Autodesk Inventor part; units mm, degrees
ref_plane "YZ Plane" through (0, 0, 0) normal (1, 0, 0) x (0, 1, 0)
ref_plane "XZ Plane" through (0, 0, 0) normal (0, 1, 0) x (-1, 0, 0)
ref_plane "XY Plane" through (0, 0, 0) normal (0, 0, 1) x (1, 0, 0)
sketch "Эскиз1" plane through (0, 0, 0) normal (0, 0, 1) x (1, 0, 0)
  line L0 (-1.0718, 4) -> (83.0251, 4)
  circle A0 centre (14.7479, 10) radius 2
  circle A1 centre (62.7479, 10) radius 2
  line L1 (-1.0718, 4) -> (-3.896, 14.54)
  line L2 (83.0251, 4) -> (83.0251, 48.71)
  line L3 (-3.896, 14.54) -> (-6.6159, 24.6909)
  line L4 (-6.6159, 24.6909) -> (83.0251, 48.71)
  dimension "d0" = 10.509
extrude "Выдавливание1" add sketch "Эскиз1" along normal blind 4
sketch "Эскиз2" plane through (83.0251, 4, 0) normal (1, 0, 0) x (0, 0, -1)
  line L0 (-4, 0) -> (-4, 44.71)
  line L1 (-4, 44.71) -> (0, 44.71)
  line L2 (0, 44.71) -> (0, 40.71)
  line L3 (0, 40.71) -> (-4, 40.71)
  line L4 (-4, 40.71) -> (-4, 44.71)
  point P0 (0, -4)
  point P1 (-4, 40.71)
  dimension "d3" = 4
  dimension "d4" = 4
extrude "Выдавливание2" add sketch "Эскиз2" along normal blind 4
pattern_linear "Прямоуг.массив1" count 6 spacing 8 along (0, -1, 0) of "Выдавливание2"
sketch "Эскиз3" plane through (0, 0, 4) normal (0, 0, 1) x (1, 0, 0)
  circle A0 centre (56.9359, 33.9549) radius 2
  line L0 (-6.6159, 24.6909) -> (-1.0718, 4)
  line L1 (-1.0718, 4) -> (83.0251, 4)
  line L2 (83.0251, 4) -> (83.0251, 4.71)
  line L3 (83.0251, 4.71) -> (87.0251, 4.71)
  line L4 (87.0251, 8.71) -> (87.0251, 4.71)
  line L5 (83.0251, 8.71) -> (87.0251, 8.71)
  line L6 (83.0251, 8.71) -> (83.0251, 12.71)
  line L7 (83.0251, 12.71) -> (87.0251, 12.71)
  line L8 (87.0251, 16.71) -> (87.0251, 12.71)
  line L9 (83.0251, 16.71) -> (87.0251, 16.71)
  line L10 (83.0251, 16.71) -> (83.0251, 20.71)
  line L11 (83.0251, 20.71) -> (87.0251, 20.71)
  line L12 (87.0251, 24.71) -> (87.0251, 20.71)
  line L13 (83.0251, 24.71) -> (87.0251, 24.71)
  line L14 (83.0251, 24.71) -> (83.0251, 28.71)
  line L15 (83.0251, 28.71) -> (87.0251, 28.71)
  line L16 (87.0251, 32.71) -> (87.0251, 28.71)
  line L17 (83.0251, 32.71) -> (87.0251, 32.71)
  line L18 (83.0251, 32.71) -> (83.0251, 36.71)
  line L19 (83.0251, 36.71) -> (87.0251, 36.71)
  line L20 (87.0251, 40.71) -> (87.0251, 36.71)
  line L21 (83.0251, 40.71) -> (87.0251, 40.71)
  line L22 (83.0251, 40.71) -> (83.0251, 44.71)
  line L23 (83.0251, 44.71) -> (87.0251, 44.71)
  line L24 (87.0251, 48.71) -> (87.0251, 44.71)
  line L25 (83.0251, 48.71) -> (87.0251, 48.71)
  line L26 (83.0251, 48.71) -> (-6.6159, 24.6909)
  circle A1 centre (62.7479, 10) radius 2
  circle A2 centre (14.7479, 10) radius 2
  circle A3 centre (37.6174, 28.7785) radius 2
  point P0 (0, 0)
  point P1 (0, 0)
extrude "Выдавливание3" cut sketch "Эскиз3" against normal blind 10 contours A0 | A3
properties part number "KB33-046-004-009 - Передняя левая боковая пластина"
Here's how the part is built. I have some questions about the finished solid (model axes, mm). A direction names the side the tool comes from. Give positions to 0.01 mm unless a question says otherwise; leave off trailing zeros. Order: outer loops, then holes, each group sorted by start corner. A loop starts at its lowest first (then second) coordinate and runs counter-clockwise, first axis right, second up. Notation, with made-up numbers: M 79.5,-8 L 137.5,-8 A17 cw 137.5,0 Z; hole C 44.5,-24.75 d8. An arc over 180 degrees is marked long. Use a Markdown table: item, result. Add a question column.
1. On a 3-axis mill with a long thin cutter (end or side, diameter ignored), from which of +Z, -Z, +X, -X, +Y, -Y can I reach the whole of each face in a straight line? I mean faces 1 (the flat face through (83.025, 35, 2)), 2 (the flat face through (85, 4.71, 2)), 3 (the flat face through (37.577, 36.532, 1.972)). Say none if no direction works.
2. Suppose I cut it at C-C (x = 36.5). List the corners of the cut face in (y, z) for me, and give its area (3 significant figures).
3. I need wall thicknesses on probe 1 along X at (y, z) = (9, 0.3); probe 2 along Y at (x, z) = (37, 2.2); probe 3 along Y at (x, z) = (38, 0.95). Which ranges of each line are inside material? Lowest first, please. Write a range as from..to.
4. If we mould it in two halves opening along Y, with no side actions, what happens to faces 4 (the flat face through (87.025, 31, 2)), 5 (the flat face through (85, 32.71, 2)), 6 (the flat face through (40, 4, 2))? For each: +Y half, -Y half, draft (parallel to the pull), parting line (faces both ways), or undercut.
5. For pin 1 Ø1.2 at (x, z) = (84.5, 2) entering from -Y; pin 2 Ø3 at (x, y) = (56.94, 33.95) entering from -Z; pin 3 Ø2 at (y, z) = (27.5, 1.5) entering from +X, each with a flat end and sliding along its axis, tell me the tip position at first contact or that it passes through.
6. Suppose I cut it at A-A (y = 10). List the corners of the cut face in (x, z) for me, and give its area (3 significant figures).
7. Suppose I cut it at D-D (y = 35). List the corners of the cut face in (x, z) for me.
8. Suppose I cut it at B-B (z = 0.95). Give the number of separate pieces and of enclosed holes in the cut face, and give its area (3 significant figures).
Results list:
| question | item | result |
|---|---|---|
| 1 | face 1 | +Z, -Z, +X |
| 1 | face 2 | +Z, -Z, +X, -Y |
| 1 | face 3 | +Z, -Z, -X, +Y |
| 2 | outline | M 4,0 L 27.12,0 L 27.12,4 L 4,4 Z; M 30.44,0 L 36.24,0 L 36.24,4 L 30.44,4 Z |
| 2 | area | 116 mm² |
| 3 | probe 1 | x = -2.41..13.02, 16.48..61.02, 64.48..83.03 |
| 3 | probe 2 | y = 4..26.88, 30.68..36.38 |
| 3 | probe 3 | y = 4..26.82, 30.74..36.65 |
| 4 | face 4 | draft |
| 4 | face 5 | undercut |
| 4 | face 6 | -Y half |
| 5 | pin 1 | stops at y = 4.71 |
| 5 | pin 2 | passes through |
| 5 | pin 3 | stops at x = 83.03 |
| 6 | outline | M -2.68,0 L 12.75,0 L 12.75,4 L -2.68,4 Z; M 16.75,0 L 60.75,0 L 60.75,4 L 16.75,4 Z; M 64.75,0 L 83.03,0 L 83.03,4 L 64.75,4 Z |
| 6 | area | 311 mm² |
| 7 | outline | M 31.86,0 L 55.23,0 L 55.23,4 L 31.86,4 Z; M 58.64,0 L 83.03,0 L 83.03,4 L 58.64,4 Z |
| 8 | separate pieces | 1 |
| 8 | enclosed holes | 4 |
| 8 | area | 2,920 mm² |
